The listing builds one solid part. Answer for the finished solid, in the listing's coordinates (mm). Face numbers are marked on the shaded views. A direction names the side the tool comes from. Coordinates: 2 decimals unless noted, no trailing zeros. Order: outer loops, then holes, each group sorted by start corner. A loop starts at its lowest first (then second) coordinate and runs counter-clockwise, first axis right, second up. Notation, with made-up numbers: (-29, -26.5) - (2, -26.5) arc R15 ccw to (2, -21.5) - close; hole circle Ø1 at (76.5, 37.25). An arc over 180 degrees is marked (long way). One line per item, written item: value. Start each with the question number.
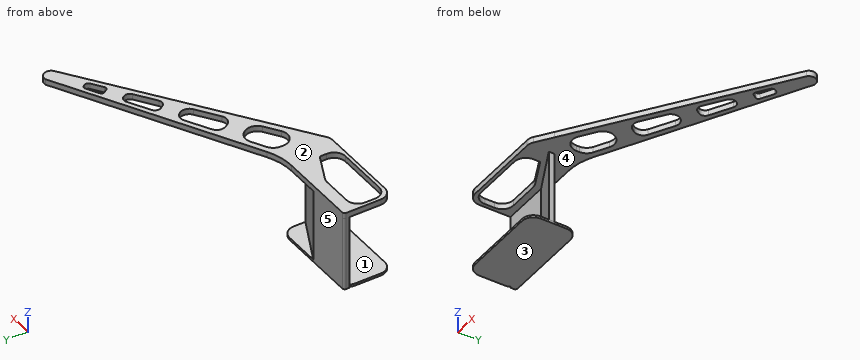
```python
from build123d import *

# Parameters (mm, degrees)
BOSS_EXTRUDE1_DEPTH = 65
BOSS_EXTRUDE2_DEPTH = 5
FILLET1_R           = 2
BOSS_EXTRUDE3_DEPTH = 2


with BuildPart() as part:
    # Sketch1 → Boss-Extrude1 (new body)
    with BuildSketch(Plane.XY):
        Polygon((141.271101362, -12.551330892), (182.617659362, -12.551330892), (224, -32.611529859), (224, -27.611529859), (182.617659362, -7.551330892), (141.271101362, -7.551330892), align=None)
    extrude(amount=BOSS_EXTRUDE1_DEPTH)

    # Sketch2 → Boss-Extrude2 (add)
    with BuildSketch(Plane.XY.offset(65)):
        with BuildLine():
            Line((141.271101362, -17.551330892), (141.271101362, -40))
            ThreePointArc((141.271101362, -40), (144.20003355, -47.071067812), (151.271101362, -50))
            Line((151.271101362, -50), (221.609244051, -50))
            ThreePointArc((221.609244051, -50), (224.616302046, -49.537169507), (227.345008414, -48.191520443))
            Line((227.345008414, -48.191520443), (241.145272825, -38.528471273))
            Line((241.145272825, -38.528471273), (404.975681683, 76.186815997))
            ThreePointArc((404.975681683, 76.186815997), (406.218347763, 83.603069448), (399.337748937, 86.636614244))
            Line((399.337748937, 86.636614244), (235.875707721, -1.555327184))
            ThreePointArc((235.875707721, -1.555327184), (224.377798441, -6.02915992), (212.134429105, -7.551330892))
            Line((212.134429105, -7.551330892), (151.271101362, -7.551330892))
            Line((151.271101362, -7.551330892), (143.271101362, -7.551330892))
            ThreePointArc((143.271101362, -7.551330892), (141.8568878, -8.13711733), (141.271101362, -9.551330892))
            Line((141.271101362, -9.551330892), (141.271101362, -17.551330892))
        make_face()
        with BuildLine():
            Line((144.446293756, -28.410757918), (144.446293756, -37.108637926))
            ThreePointArc((144.446293756, -37.108637926), (147.375225944, -44.179705738), (154.446293756, -47.108637926))
            Line((154.446293756, -47.108637926), (200, -47.108637926))
            ThreePointArc((200, -47.108637926), (207.071067812, -44.179705738), (210, -37.108637926))
            Line((210, -37.108637926), (210, -30.978450453))
            Line((210, -30.978450453), (185.025223493, -19.345830567))
            ThreePointArc((185.025223493, -19.345830567), (182.965268196, -18.647324262), (180.803009367, -18.410757918))
            Line((180.803009367, -18.410757918), (154.446293756, -18.410757918))
            ThreePointArc((154.446293756, -18.410757918), (147.375225944, -21.339690106), (144.446293756, -28.410757918))
        make_face(mode=Mode.SUBTRACT)
        with BuildLine():
            Line((251.535159303, -24.247899123), (263.816616141, -15.81719868))
            ThreePointArc((263.816616141, -15.81719868), (267.988692729, -9.400624773), (266.401593453, -1.913318204))
            Line((266.401593453, -1.913318204), (265.970804926, -1.28576528))
            ThreePointArc((265.970804926, -1.28576528), (260.036959634, 2.784182062), (252.906809883, 1.816733956))
            Line((252.906809883, 1.816733956), (241.056141572, -4.701800674))
            ThreePointArc((241.056141572, -4.701800674), (237.267698036, -8.374334113), (235.875707721, -13.463751492))
            Line((235.875707721, -13.463751492), (235.875707721, -16.003470229))
            ThreePointArc((235.875707721, -16.003470229), (241.21708753, -24.852044007), (251.535159303, -24.247899123))
        make_face(mode=Mode.SUBTRACT)
        with BuildLine():
            Line((378.147749465, 66.305107432), (377.492648494, 67.259428411))
            ThreePointArc((377.492648494, 67.259428411), (375.712494906, 68.480412613), (373.573449981, 68.190178181))
            Line((373.573449981, 68.190178181), (363.266327618, 62.520680707))
            ThreePointArc((363.266327618, 62.520680707), (362.038869424, 60.907838903), (362.410111932, 58.915330107))
            Line((362.410111932, 58.915330107), (364.285761939, 56.182969403))
            ThreePointArc((364.285761939, 56.182969403), (365.889905415, 55.139950256), (367.761732058, 55.536725075))
            Line((367.761732058, 55.536725075), (377.372256271, 62.133943289))
            ThreePointArc((377.372256271, 62.133943289), (378.623879248, 64.058915461), (378.147749465, 66.305107432))
        make_face(mode=Mode.SUBTRACT)
        with BuildLine():
            Line((280.18309969, 4.514751946), (278.736858234, 6.621570014))
            ThreePointArc((278.736858234, 6.621570014), (277.623130083, 12.599093755), (281.305500525, 17.437619191))
            Line((281.305500525, 17.437619191), (301.361850744, 28.469759713))
            ThreePointArc((301.361850744, 28.469759713), (306.709465178, 29.195349043), (311.159851794, 26.142887908))
            Line((311.159851794, 26.142887908), (311.329646681, 25.895538523))
            ThreePointArc((311.329646681, 25.895538523), (312.519971137, 20.280058597), (309.390913697, 15.467628166))
            Line((309.390913697, 15.467628166), (290.611010047, 2.576018962))
            ThreePointArc((290.611010047, 2.576018962), (284.995530121, 1.385694505), (280.18309969, 4.514751946))
        make_face(mode=Mode.SUBTRACT)
        with BuildLine():
            Line((325.111152918, 32.323608673), (323.645737546, 34.45835842))
            ThreePointArc((323.645737546, 34.45835842), (322.903252531, 38.443376012), (325.358168918, 41.66905962))
            Line((325.358168918, 41.66905962), (343.672425355, 51.742931547))
            ThreePointArc((343.672425355, 51.742931547), (347.237500231, 52.2266556), (350.204422877, 50.191681929))
            Line((350.204422877, 50.191681929), (350.504255702, 49.754899253))
            ThreePointArc((350.504255702, 49.754899253), (351.297805339, 46.011245969), (349.211767046, 42.802959015))
            Line((349.211767046, 42.802959015), (332.063093156, 31.031120017))
            ThreePointArc((332.063093156, 31.031120017), (328.319439871, 30.237570379), (325.111152918, 32.323608673))
        make_face(mode=Mode.SUBTRACT)
    extrude(amount=BOSS_EXTRUDE2_DEPTH)

    # Fillet1
    fillet1_edges = [part.edges().sort_by_distance(p)[0] for p in [
        (141.271101362, -7.551330892, 32.5),
    ]]
    fillet(fillet1_edges, radius=FILLET1_R)

    # Sketch3 → Boss-Extrude3 (add)
    with BuildSketch(Plane(origin=(0, 0, 0), x_dir=(-1, 0, 0), z_dir=(0, 0, -1))):
        with BuildLine():
            Line((-141.271101362, -26.275665446), (-141.271101362, -40.012233887))
            ThreePointArc((-141.271101362, -40.012233887), (-144.20003355, -47.083301699), (-151.271101362, -50.012233887))
            Line((-151.271101362, -50.012233887), (-214.616302046, -50.012233887))
            ThreePointArc((-214.616302046, -50.012233887), (-221.687369858, -47.083301699), (-224.616302046, -40.012233887))
            Line((-224.616302046, -40.012233887), (-224.616302046, -26.275665446))
            Line((-224.616302046, -26.275665446), (-224.616302193, -17.551331061))
            ThreePointArc((-224.616302193, -17.551331061), (-221.687370065, -10.48026314), (-214.616302193, -7.551330892))
            Line((-214.616302193, -7.551330892), (-151.271101362, -7.551330892))
            ThreePointArc((-151.271101362, -7.551330892), (-144.20003355, -10.48026308), (-141.271101362, -17.551330892))
            Line((-141.271101362, -17.551330892), (-141.271101362, -26.275665446))
        make_face()
    extrude(amount=-BOSS_EXTRUDE3_DEPTH)


solid = part.part
```
(1) Consider probe 1 along Z at (x, y) = (327, 27); probe 2 along Y at (x, z) = (309.5, 65.5); probe 3 along Y at (x, z) = (169.5, 36.5). Determine where each line is inside the solid, lowest interval first.
(2) For the marked faces 1 and 2, determine the directions among +Z, -Z, +X, -X, +Y, -Y from which every point of the face is accessible in a straight line to the end or side of a thin tool.
(3) The part is cut by section A-A on z = 18. Determine the outline of the cut face in (x, y).
(4) Flat-ended cylindrical pins translate along their axes: pin 1 Ø5.5 at (y, z) = (-30, 27) entering from +X; pin 2 Ø2.5 at (y, z) = (-31.5, 68.5) entering from +X; pin 3 Ø1 at (y, z) = (-23.5, 0.5) entering from +X. Find the tip coordinate at first contact, or state that the pin passes through.
(5) The part is cut by section B-B on x = 230. Determine the outline of the cut face in (y, z).
(6) For a pull along Z with two mould halves and no side action, classify the marked faces 3, 4 and 5 as pulls with the +Z half, pulls with the -Z half, needs draft (parallel to the pull), parting line crosses it, or undercut.
Completed:
1. probe 1: z = 65 to 70
1. probe 2: y = 9.33 to 15.54, 27.88 to 38.17
1. probe 3: y = -12.55 to -7.55
2. face 1: none
2. face 2: +Z, +X, -X, +Y, -Y
3. outline: (141.27, -12.55) - (182.62, -12.55) - (224, -32.61) - (224, -27.61) - (182.62, -7.55) - (143.27, -7.55) arc R2 ccw to (141.27, -9.55) - close
4. pin 1: stops at x = 224
4. pin 2: stops at x = 252.97
4. pin 3: stops at x = 224.62
5. outline: (-46.33, 65) - (-4.25, 65) - (-4.25, 70) - (-46.33, 70) - close
6. face 3: pulls with the -Z half
6. face 4: undercut
6. face 5: needs draft
